For this review, take the finished solid that the model builds, in its own axes (mm). Face numbers are marked on the shaded views. Coordinates: 2 decimals unless noted, no trailing zeros. Order: outer loops, then holes, each group sorted by start corner. A loop starts at its lowest first (then second) coordinate and runs counter-clockwise, first axis right, second up. Notation, with made-up numbers: (53, 22) -> (83, 22) arc R24 cw to (83, 43) -> close; hole circle Ø7 at (66, 71). An arc over 180 degrees is marked (long way). Answer as a JSON object with one key per item and string values. Group by question number.
1) Add section A-A, the plane x = -15.9. Write out the cut boundary in (y, z) (3 decimals), then the cut area to 3 significant figures.
2) Add section C-C, the plane z = 0. Write out the cut boundary in (x, y), then the cut area to 3 significant figures.
3) Wall thickness on L1, parallel to Z at x = 15.9, y = 8.75; L2, parallel to Z at x = -23.55, y = 2.25; L3, parallel to X at y = 5.5, z = -25.5: over which ranges is each line inside the solid? List them lowest first.
4) For pin 1 (0.8 mm diameter, centred on y = 2, z = -26, fed in from -X); pin 2 (5 mm diameter, centred on x = 21, y = 9.5, fed in from +Z); pin 3 (2 mm diameter, centred on x = -24.5, y = 6.5, fed in from -Z), all flat-tipped, find the tip position at first contact; note any pin that passes through.
5) Add section B-B, the plane y = 4. Count the separate pieces of the cut face and the enclosed holes in it, then the cut area to 3 significant figures.
6) Draft analysis for pull direction X (two halves, no side actions). For the marked faces 1, 2, 3 and 4, state which applies: +X half, -X half, draft (parallel to the pull), parting line (faces both ways), or undercut.
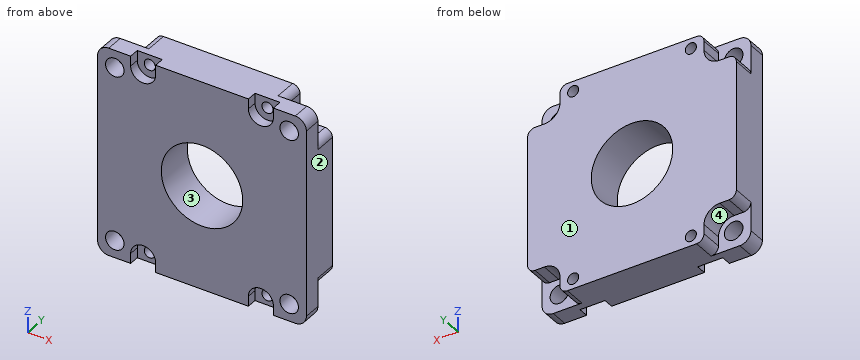
from build123d import *

# Parameters (mm, degrees)
SKETCH003_R          = 5.5
PAD002_DEPTH         = 6
SKETCH_R             = 5.5
PAD_DEPTH            = 5
SKETCH005_R          = 19.05
SKETCH005_R_2        = 5.5
PAD004_DEPTH         = 1.1
SKETCH006_R          = 2.5
POCKET_DEPTH         = 11.001
SKETCH007_R          = 1.5
POCKET001_DEPTH      = 12.101
POCKET004_DEPTH      = 3
SKETCH018_R          = 11
POCKET009_DEPTH      = 11
POCKET009_FACE32_R   = 2.5
POCKET009_FACE32_R_2 = 19.05
POCKET014_DEPTH      = 0.25
POCKET014_FACE62_R   = 19.05
POCKET014_FACE62_R_2 = 5.5
POCKET021_DEPTH      = 1.35


with BuildPart() as part:
    # Sketch003 → Pad002 (new body)
    with BuildSketch(Plane(origin=(0, 5, 0), x_dir=(1, 0, 0), z_dir=(0, 1, 0))):
        with BuildLine():
            Line((-26.2, 19.45), (-23.7, 19.45))
            ThreePointArc((-23.7, 19.45), (-20.694796, 20.694796), (-19.45, 23.7))
            Line((-19.45, 23.7), (-19.45, 26.2))
            ThreePointArc((-17.45, 28.2), (-18.864214, 27.614214), (-19.45, 26.2))
            Line((-17.45, 28.2), (17.45, 28.2))
            ThreePointArc((19.45, 26.2), (18.864214, 27.614214), (17.45, 28.2))
            Line((19.45, 26.2), (19.45, 23.7))
            ThreePointArc((19.45, 23.7), (20.694796, 20.694796), (23.7, 19.45))
            Line((23.7, 19.45), (26.2, 19.45))
            ThreePointArc((28.2, 17.45), (27.614214, 18.864214), (26.2, 19.45))
            Line((28.2, 17.45), (28.2, -17.45))
            ThreePointArc((26.2, -19.45), (27.614214, -18.864214), (28.2, -17.45))
            Line((23.7, -19.45), (26.2, -19.45))
            ThreePointArc((23.7, -19.45), (20.694796, -20.694796), (19.45, -23.7))
            Line((19.45, -26.2), (19.45, -23.7))
            ThreePointArc((17.45, -28.2), (18.864214, -27.614214), (19.45, -26.2))
            Line((-17.45, -28.2), (17.45, -28.2))
            ThreePointArc((-19.45, -26.2), (-18.864214, -27.614214), (-17.45, -28.2))
            Line((-19.45, -26.2), (-19.45, -23.7))
            ThreePointArc((-19.45, -23.7), (-20.694796, -20.694796), (-23.7, -19.45))
            Line((-26.2, -19.45), (-23.7, -19.45))
            ThreePointArc((-28.2, -17.45), (-27.614214, -18.864214), (-26.2, -19.45))
            Line((-28.2, 17.45), (-28.2, -17.45))
            ThreePointArc((-26.2, 19.45), (-27.614214, 18.864214), (-28.2, 17.45))
        make_face()
        Circle(SKETCH003_R, mode=Mode.SUBTRACT)
    extrude(amount=PAD002_DEPTH)

    # Sketch (on Face26 of Pad002) → Pad (join)
    with BuildSketch(Plane.XZ.offset(-5)):
        with BuildLine():
            Line((-28.2, 25.2), (-28.2, -25.2))
            ThreePointArc((-28.2, -25.2), (-27.32132, -27.32132), (-25.2, -28.2))
            Line((-25.2, -28.2), (25.2, -28.2))
            ThreePointArc((25.2, -28.2), (27.32132, -27.32132), (28.2, -25.2))
            Line((28.2, 25.2), (28.2, -25.2))
            ThreePointArc((28.2, 25.2), (27.32132, 27.32132), (25.2, 28.2))
            Line((-25.2, 28.2), (25.2, 28.2))
            ThreePointArc((-25.2, 28.2), (-27.32132, 27.32132), (-28.2, 25.2))
        make_face()
        Circle(SKETCH_R, mode=Mode.SUBTRACT)
    extrude(amount=PAD_DEPTH)

    # Sketch005 (on Face33 of Pad) → Pad004 (join)
    with BuildSketch(Plane.XZ):
        Circle(SKETCH005_R)
        Circle(SKETCH005_R_2, mode=Mode.SUBTRACT)
    extrude(amount=PAD004_DEPTH)

    # Sketch006 (on Face33 of Pad004) → Pocket (cut, through all)
    with BuildSketch(Plane.XZ):
        with Locations((-23.55, 23.55)):
            Circle(SKETCH006_R)
        with Locations((23.55, 23.55)):
            Circle(SKETCH006_R)
        with Locations((23.55, -23.55)):
            Circle(SKETCH006_R)
        with Locations((-23.55, -23.55)):
            Circle(SKETCH006_R)
    extrude(amount=-POCKET_DEPTH, mode=Mode.SUBTRACT)

    # Sketch007 (on Face5 of Pocket) → Pocket001 (cut, through all)
    with BuildSketch(Plane(origin=(0, 11, 0), x_dir=(1, 0, 0), z_dir=(0, 1, 0))):
        with Locations((-15.9, 25.5)):
            Circle(SKETCH007_R)
        with Locations((15.9, 25.5)):
            Circle(SKETCH007_R)
        with Locations((-15.9, -25.5)):
            Circle(SKETCH007_R)
        with Locations((15.9, -25.5)):
            Circle(SKETCH007_R)
    extrude(amount=-POCKET001_DEPTH, mode=Mode.SUBTRACT)

    # Sketch012 (on Face38 of Pocket001) → Pocket004 (cut)
    with BuildSketch(Plane.XZ):
        with BuildLine():
            Line((-19.275, -25.5), (-19.275, -30.5))
            Line((-19.275, -30.5), (-12.525, -30.5))
            Line((-12.525, -30.5), (-12.525, -25.5))
            ThreePointArc((-12.525, -25.5), (-15.9, -22.125), (-19.275, -25.5))
        make_face()
        with BuildLine():
            Line((12.525, -25.5), (12.525, -30.5))
            Line((12.525, -30.5), (19.275, -30.5))
            Line((19.275, -30.5), (19.275, -25.5))
            ThreePointArc((19.275, -25.5), (15.9, -22.125), (12.525, -25.5))
        make_face()
        with BuildLine():
            Line((-19.275, 25.5), (-19.275, 30.5))
            Line((-19.275, 30.5), (-12.525, 30.5))
            Line((-12.525, 30.5), (-12.525, 25.5))
            ThreePointArc((-19.275, 25.5), (-15.9, 22.125), (-12.525, 25.5))
        make_face()
        with BuildLine():
            Line((12.525, 25.5), (12.525, 30.5))
            Line((12.525, 30.5), (19.275, 30.5))
            Line((19.275, 30.5), (19.275, 25.5))
            ThreePointArc((12.525, 25.5), (15.9, 22.125), (19.275, 25.5))
        make_face()
    extrude(amount=-POCKET004_DEPTH, mode=Mode.SUBTRACT)

    # Sketch018 (on Face5 of Pocket004) → Pocket009 (cut)
    with BuildSketch(Plane(origin=(0, 11, 0), x_dir=(1, 0, 0), z_dir=(0, 1, 0))):
        Circle(SKETCH018_R)
    extrude(amount=-POCKET009_DEPTH, mode=Mode.SUBTRACT)

    # Pocket009 Face32 → Pocket014 (cut)
    with BuildSketch(Plane(origin=(0, 0, 0), x_dir=(-1, 0, 0), z_dir=(0, -1, 0))):
        with BuildLine():
            Line((19.275, -28.2), (25.2, -28.2))
            ThreePointArc((25.2, -28.2), (27.32132, -27.32132), (28.2, -25.2))
            Line((28.2, -25.2), (28.2, 25.2))
            ThreePointArc((28.2, 25.2), (27.32132, 27.32132), (25.2, 28.2))
            Line((25.2, 28.2), (19.275, 28.2))
            Line((19.275, 28.2), (19.275, 25.5))
            ThreePointArc((19.275, 25.5), (15.9, 22.125), (12.525, 25.5))
            Line((12.525, 25.5), (12.525, 28.2))
            Line((12.525, 28.2), (-12.525, 28.2))
            Line((-12.525, 28.2), (-12.525, 25.5))
            ThreePointArc((-12.525, 25.5), (-15.9, 22.125), (-19.275, 25.5))
            Line((-19.275, 25.5), (-19.275, 28.2))
            Line((-19.275, 28.2), (-25.2, 28.2))
            ThreePointArc((-25.2, 28.2), (-27.32132, 27.32132), (-28.2, 25.2))
            Line((-28.2, 25.2), (-28.2, -25.2))
            ThreePointArc((-28.2, -25.2), (-27.32132, -27.32132), (-25.2, -28.2))
            Line((-25.2, -28.2), (-19.275, -28.2))
            Line((-19.275, -28.2), (-19.275, -25.5))
            ThreePointArc((-19.275, -25.5), (-15.9, -22.125), (-12.525, -25.5))
            Line((-12.525, -25.5), (-12.525, -28.2))
            Line((-12.525, -28.2), (12.525, -28.2))
            Line((12.525, -28.2), (12.525, -25.5))
            ThreePointArc((12.525, -25.5), (15.9, -22.125), (19.275, -25.5))
            Line((19.275, -25.5), (19.275, -28.2))
        make_face()
        with Locations((23.55, -23.55)):
            Circle(POCKET009_FACE32_R, mode=Mode.SUBTRACT)
        with Locations((23.55, 23.55)):
            Circle(POCKET009_FACE32_R, mode=Mode.SUBTRACT)
        Circle(POCKET009_FACE32_R_2, mode=Mode.SUBTRACT)
        with Locations((-23.55, -23.55)):
            Circle(POCKET009_FACE32_R, mode=Mode.SUBTRACT)
        with Locations((-23.55, 23.55)):
            Circle(POCKET009_FACE32_R, mode=Mode.SUBTRACT)
    extrude(amount=-POCKET014_DEPTH, mode=Mode.SUBTRACT)

    # Pocket014 Face62 → Pocket021 (cut)
    with BuildSketch(Plane(origin=(0, -1.1, 0), x_dir=(-1, 0, 0), z_dir=(0, -1, 0))):
        Circle(POCKET014_FACE62_R)
        Circle(POCKET014_FACE62_R_2, mode=Mode.SUBTRACT)
    extrude(amount=-POCKET021_DEPTH, mode=Mode.SUBTRACT)


solid = part.part
Output values:
{
 "1": {"outline": "(0.25, -22.125) -> (3, -22.125) -> (3, -24) -> (11, -24) -> (11, 24) -> (3, 24) -> (3, 22.125) -> (0.25, 22.125) -> close; (3, -28.2) -> (11, -28.2) -> (11, -27) -> (3, -27) -> close; (3, 27) -> (11, 27) -> (11, 28.2) -> (3, 28.2) -> close", "area": "525 mm²"},
 "2": {"outline": "(-28.2, 0.25) -> (-11, 0.25) -> (-11, 11) -> (-28.2, 11) -> close; (11, 0.25) -> (28.2, 0.25) -> (28.2, 11) -> (11, 11) -> close", "area": "370 mm²"},
 "3": {"L1": "z = -28.2 to -27, -24 to 24, 27 to 28.2", "L2": "z = -28.2 to -26.05, -21.05 to 21.05, 26.05 to 28.2", "L3": "x = -19.45 to -17.4, -14.4 to 14.4, 17.4 to 19.45"},
 "4": {"pin 1": "stops at x = -28.17", "pin 2": "stops at z = 27.9", "pin 3": "stops at z = -19.45"},
 "5": {"separate pieces": "1", "enclosed holes": "9", "area": "2,690 mm²"},
 "6": {"face 1": "draft", "face 2": "+X half", "face 3": "undercut", "face 4": "-X half"}
}
